```python
from build123d import *

# Parameters (mm, degrees)
SKETCH2_R           = 6.8
SKETCH2_R_2         = 1
BOSS_EXTRUDE1_DEPTH = 3


with BuildPart() as part:
    # Sketch1 → Revolve1 (revolve)
    with BuildSketch(Plane.XY):
        Polygon((11, 12.28125), (6.8, 12.28125), (6.8, 9.28125), (6, 9.28125), (6, -32.71875), (11, -32.71875), align=None)
    revolve(axis=Axis((0, 17.71875, 0), (0, -1, 0)))

    # Sketch2 → Boss-Extrude1 (add)
    with BuildSketch(Plane.XZ.offset(32.71875)):
        with BuildLine():
            Line((-23.5, -2.598076211), (9.5, -21.650635095))
            ThreePointArc((9.5, -21.650635095), (12.5, -21.650635095), (14, -19.052558883))
            Line((14, -19.052558883), (14, 19.052558883))
            ThreePointArc((14, 19.052558883), (12.5, 21.650635095), (9.5, 21.650635095))
            Line((9.5, 21.650635095), (-23.5, 2.598076211))
            ThreePointArc((-23.5, 2.598076211), (-25, 0), (-23.5, -2.598076211))
        make_face()
        Circle(SKETCH2_R, mode=Mode.SUBTRACT)
        with Locations((11.65, 20.178391908)):
            Circle(SKETCH2_R_2, mode=Mode.SUBTRACT)
        with Locations((-23.3, 0)):
            Circle(SKETCH2_R_2, mode=Mode.SUBTRACT)
        with Locations((11.65, -20.178391908)):
            Circle(SKETCH2_R_2, mode=Mode.SUBTRACT)
    extrude(amount=BOSS_EXTRUDE1_DEPTH)


solid = part.part
```
The listing builds one solid part. Answer for the finished solid, in the listing's coordinates (mm). A direction names the side the tool comes from. Round coordinates to 2 decimals unless told otherwise and drop trailing zeros. Loops run counter-clockwise (first coordinate to the right, second up) from the corner with the lowest first, then second, coordinate; pieces in that order, holes last. Notation, with made-up numbers: (26.5, -17) - (36.5, -17) arc R37 ccw to (36.5, 21) - close; hole circle Ø2 at (13.25, 43). An arc over 180 degrees is marked (long way). Return JSON: item names as keys, results as strings. Group by question number.
1. The part is cut by section B-B on x = 2.5. Determine the outline of the cut face in (y, z).
2. The part is cut by section C-C on y = -7. Determine the outline of the cut face in (x, z).
3. The part is cut by section A-A on z = 0. Determine the outline of the cut face in (x, y).
4. Consider probe 1 along Z at (x, y) = (0, 11); probe 2 along Z at (x, y) = (11, -34); probe 3 along Y at (x, z) = (11.5, 0.5). Determine where each line is inside the solid, lowest interval first.
5. The mould has two halves that part along Z. Classify faces 4 (the flat face through (-6.769, -34.198, 12.258)), 5 (the cylindrical face through (-1.47, 10.76, -6.64)), 6 (the cylindrical face through (-2.38, -9.9, -10.74)): pulls with the +Z half, pulls with the -Z half, needs draft (parallel to the pull), parting line crosses it, or undercut.
6. Which of the six approach directions +Z, -Z, +X, -X, +Y, -Y give full straight-line access (tool end or side, diameter ignored) to faces 1 (the flat face through (-4, -32.719, -5)), 2 (the flat face through (-6, -35.719, 5)), 3 (the flat face through (-11, -32.719, -2))?
7. Each of these flat-tipped pins is pushed along its axis until it touches: P1, Ø6, axis at y = -3.5, z = 6.5, coming from the -X side; P2, Ø3, axis at y = -14.5, z = -2, coming from the +X side; P3, Ø7, axis at x = 1, z = -3, coming from the -Y side. Where does it stop, or does it pass through?
8. The part is cut by section D-D on x = 11.65. Determine the outline of the cut face in (y, z).
Resolved:
{
 "1": {"outline": "(-35.72, -17.61) - (-32.72, -17.61) - (-32.72, -10.71) - (12.28, -10.71) - (12.28, -6.32) - (9.28, -6.32) - (9.28, -5.45) - (-32.72, -5.45) - (-32.72, -6.32) - (-35.72, -6.32) - close; (-35.72, 6.32) - (-32.72, 6.32) - (-32.72, 5.45) - (9.28, 5.45) - (9.28, 6.32) - (12.28, 6.32) - (12.28, 10.71) - (-32.72, 10.71) - (-32.72, 17.61) - (-35.72, 17.61) - close"},
 "2": {"outline": "circle Ø22 at (0, 0); hole circle Ø12 at (0, 0)"},
 "3": {"outline": "(-25, -35.72) - (-24.3, -35.72) - (-24.3, -32.72) - (-25, -32.72) - close; (-22.3, -35.72) - (-6.8, -35.72) - (-6.8, -32.72) - (-6, -32.72) - (-6, 9.28) - (-6.8, 9.28) - (-6.8, 12.28) - (-11, 12.28) - (-11, -32.72) - (-22.3, -32.72) - close; (6, -32.72) - (6.8, -32.72) - (6.8, -35.72) - (14, -35.72) - (14, -32.72) - (11, -32.72) - (11, 12.28) - (6.8, 12.28) - (6.8, 9.28) - (6, 9.28) - close"},
 "4": {"probe 1": "z = -11 to -6.8, 6.8 to 11", "probe 2": "z = -22.05 to -20.94, -19.42 to 19.42, 20.94 to 22.05", "probe 3": "y = -35.72 to -32.72"},
 "5": {"face 4": "pulls with the +Z half", "face 5": "undercut", "face 6": "parting line crosses it"},
 "6": {"face 1": "-Y", "face 2": "+Z, -Z, +X, -X, -Y", "face 3": "+Y"},
 "7": {"P1": "stops at x = -10.43", "P2": "stops at x = 10.99", "P3": "stops at y = -32.72"},
 "8": {"outline": "(-35.72, -21.98) - (-32.72, -21.98) - (-32.72, -21.18) - (-35.72, -21.18) - close; (-35.72, -19.18) - (-32.72, -19.18) - (-32.72, 19.18) - (-35.72, 19.18) - close; (-35.72, 21.18) - (-32.72, 21.18) - (-32.72, 21.98) - (-35.72, 21.98) - close"}
}
